Autodesk Fusion 360 part; units mm, degrees
sketch "Sketch1" plane through (0, 0, 0) normal (0, 0, 1) x (1, 0, 0)
  line L0 (0, 0) -> (6, 0)
  line L1 (6, 0) -> (6, 6)
  line L2 (6, 6) -> (0, 6)
  line L3 (0, 6) -> (0, 0)
  line L4 (6, 0) -> (8, 0)
  line L5 (8, 0) -> (8, 24.5)
  line L6 (8, 24.5) -> (6, 24.5)
  line L7 (6, 24.5) -> (6, 0)
  line L8 (6, 24.5) -> (17.5, 24.5)
  line L9 (17.5, 24.5) -> (17.5, 22.5)
  line L10 (17.5, 22.5) -> (6, 22.5)
  line L11 (6, 22.5) -> (6, 24.5)
  line L12 (29, 6) -> (35, 6)
  line L13 (17.5, 22.5) -> (29, 22.5)
  line L14 (29, 0) -> (29, 6)
  line L15 (35, 6) -> (35, 0)
  line L16 (29, 24.5) -> (29, 0)
  line L17 (27, 24.5) -> (29, 24.5)
  line L18 (17.5, 24.5) -> (17.5, 22.5)
  line L19 (29, 22.5) -> (29, 24.5)
  line L20 (35, 0) -> (29, 0)
  line L21 (29, 24.5) -> (17.5, 24.5)
  line L22 (27, 0) -> (27, 24.5)
  line L23 (29, 0) -> (27, 0)
  point P0 (35, 0)
  dimension "d1" = 6
  dimension "d2" = 6
  dimension "d3" = 2
  dimension "d4" = 24.5
  dimension "d5" = 11.5
  dimension "d6" = 2
extrude "Extrude1" add sketch "Sketch1" along normal blind 3 and the other way blind 3 contours L0 L1 L2 L3 L7 | L12 L14 L15 L16 L20 makes body 1 at (31, 6, -1) makes body 2 at (0, 2, 1)
extrude "Extrude2" add sketch "Sketch1" along normal blind 1.5 and the other way blind 1.5 contours L1 L4 L5 L7 L10 | L5 L6 L7 L8 L10 L11 | L5 L8 L9 L10 L18 | L9 L13 L18 L21 L22 | L13 L16 L17 L19 L21 L22 | L13 L14 L16 L22 L23 bodies 1 2
sketch "Sketch3" plane through (0, 6, 0) normal (0, 1, 0) x (-1, 0, 0)
  line L0 (0, -3) -> (0, 3)
  line L1 (0, 3) -> (-6, 3)
  line L2 (-6, 3) -> (-6, 1.5)
  line L3 (-6, 1.5) -> (-6, -1.5)
  line L4 (-6, -1.5) -> (-6, -3)
  line L5 (-6, -3) -> (0, -3)
  circle A0 centre (-3, 0) radius 1.5
  circle A1 centre (-32, 0) radius 1.5
  line L6 (-35, -3) -> (-35, 3)
  line L7 (-29, -3) -> (-35, -3)
  dimension "d16" = 3
  dimension "d17" = 3
  dimension "d18" = 3
  dimension "d19" = 3
  dimension "d20" = 3
  dimension "d21" = 3
extrude "Extrude3" cut sketch "Sketch3" against normal blind 11 contours A0 | A1 bodies 1
extrude "Extrude4" add 1 faces at (27.6667, 9.5, 1.5) along direction (0, 0, 1) up to surface (1.5 mm away) on bodies 1 bodies 1
For this review, take the finished solid that the model builds, in its own axes (mm). A direction names the side the tool comes from. Give positions to 0.01 mm unless a question says otherwise; leave off trailing zeros. Write each loop counter-clockwise with the first axis right and the second up, starting at its lowest first coordinate (ties: lowest second). Pieces come first, ordered by that corner, then holes. Notation, with made-up numbers: (-40, 29.25) -> (16, 29.25) arc R29 cw to (16, 67.25) -> close; hole circle Ø9 at (-39.75, 11). An arc over 180 degrees is marked (long way). Use CSV: the item, a comma, the result in double quotes.
Q1. Mouldability with a two-part tool opening along Z and no side actions: class faces 1 (the face through (1.57, 3.04, 0.45)), 2 (the face through (3, 3, -3)), 3 (the face through (33.2, 3, -0.9)), 4 (the face through (0, 3, 0)) as pulls with the +Z half, pulls with the -Z half, needs draft (parallel to the pull), parting line crosses it, or undercut.
Conclusion:
face 1,"undercut"
face 2,"pulls with the -Z half"
face 3,"undercut"
face 4,"needs draft"
Q2. Tool access review of faces 5 (the face through (16, 23, -1.5)), 6 (the face through (29, 15, 1)), 7 (the face through (8, 11, 1)): name each direction out of +Z, -Z, +X, -X, +Y, -Y from which nothing blocks a thin tool from reaching the whole face with its end or side.
Conclusion:
face 5,"-Z, +Y, -Y"
face 6,"+Z, -Z, +X, +Y"
face 7,"+Z, -Z, -Y"
Q3. For P1, Ø3, axis at y = 15, z = 0.5, coming from the -X side; P2, Ø1.5, axis at y = 17, z = 2.5, coming from the +X side; P3, Ø6, axis at x = 4, y = 16, coming from the -Z side, all flat-tipped, find the tip position at first contact; note any pin that passes through.
Conclusion:
P1,"x = 6"
P2,"x = 29"
P3,"z = -1.5"
Q4. Take a section at C-C, the plane z = 0. Write out the cut boundary in (x, y), then the cut area to 3 significant figures.
Conclusion:
outline,"(0, 0) -> (1.5, 0) -> (1.5, 6) -> (0, 6) -> close; (4.5, 0) -> (8, 0) -> (8, 22.5) -> (27, 22.5) -> (27, 0) -> (30.5, 0) -> (30.5, 6) -> (29, 6) -> (29, 24.5) -> (6, 24.5) -> (6, 6) -> (4.5, 6) -> close; (33.5, 0) -> (35, 0) -> (35, 6) -> (33.5, 6) -> close"
area,"172 mm2"
Q5. Take a section at D-D, the plane x = 9.5. Write out the cut boundary in (y, z), then the cut area to 3 significant figures.
Conclusion:
outline,"(22.5, -1.5) -> (24.5, -1.5) -> (24.5, 3) -> (22.5, 3) -> close"
area,"9.00 mm2"
Q6. Take a section at B-B, the plane z = -2.25. Write out the cut boundary in (x, y), then the cut area to 3 significant figures.
Conclusion:
outline,"(0, 0) -> (6, 0) -> (6, 6) -> (0, 6) -> close; (29, 0) -> (35, 0) -> (35, 6) -> (29, 6) -> close"
area,"72.0 mm2"
Q7. Take a section at A-A, the plane y = 19.25. Write out the cut boundary in (x, z).
Conclusion:
outline,"(6, -1.5) -> (8, -1.5) -> (8, 3) -> (6, 3) -> close; (27, -1.5) -> (29, -1.5) -> (29, 3) -> (27, 3) -> close"
Q8. To check wall thickness, follow probe 1 along Z at (x, y) = (32, 3.35); probe 2 along X at (y, z) = (4.5, 1.05); probe 3 along Y at (x, z) = (16, 0.85). State the ranges of each line that lie inside material, in increasing order. Write a range as [from, to].
Conclusion:
probe 1,"[-3, -1.5], [1.5, 3]"
probe 2,"[0, 1.93], [4.07, 8], [27, 30.93], [33.07, 35]"
probe 3,"[22.5, 24.5]"
